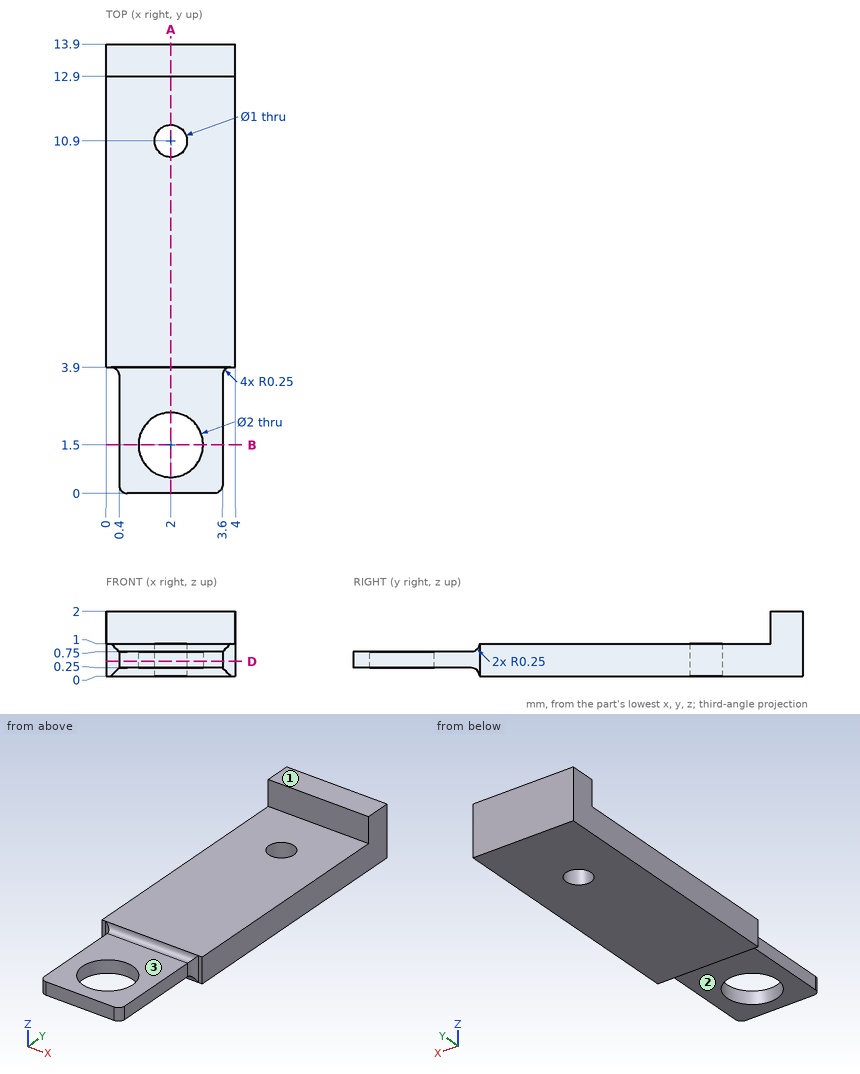
Part print with two shaded views. Sizes in mm from the minimum x, y, z corner. A direction names the side the tool comes from. Round coordinates to 2 decimals unless told otherwise and drop trailing zeros. Order: outer loops, then holes, each group sorted by start corner. A loop starts at its lowest first (then second) coordinate and runs counter-clockwise, first axis right, second up. Notation, with made-up numbers: M 51.5,-13 L 82.5,-13 A17 ccw 82.5,15 Z; hole C -29.75,87 d5. An arc over 180 degrees is marked long. Use CSV: the item, a comma, the result in double quotes. Start each with the question number.
(1) Flat gauge pins, fed straight in: P1, Ø1.2, axis at x = 2, y = 10.5, coming from the +Z side; P2, Ø1, axis at x = 3, y = 1.5, coming from the +Z side; P3, Ø1, axis at x = 1.5, y = 1, coming from the -Z side. Where does each tip first touch, or does it go through?
(2) Cut at A-A on x = 2. State how many separate pieces and enclosed holes the cut face has, then the cut area to 3 significant figures.
(3) Tool access for the marked faces 1, 2 and 3: list every direction of +Z, -Z, +X, -X, +Y, -Y with a clear straight run to the whole face (end or side of a thin tool).
(4) Drill centre lines: probe 1 along Y at (x, z) = (2, 0.65); probe 2 along Z at (x, y) = (3.15, 7); probe 3 along Z at (x, y) = (3.2, 3). Where is each one in solid material? Low to high.
(5) Cut at D-D on z = 0.45. List the corners of the cut face in (x, y).
(6) Cut at B-B on y = 1.5. List the corners of the cut face in (x, z).
Findings:
1,P1,"stops at z = 1"
1,P2,"stops at z = 0.75"
1,P3,"stops at z = 0.25"
2,separate pieces,"3"
2,enclosed holes,"0"
2,area,"11.0 mm^2"
3,face 1,"+Z, +X, -X, +Y, -Y"
3,face 2,"-Z, +X, -X, -Y"
3,face 3,"+Z, +X, -X, -Y"
4,probe 1,"y = 0 to 0.5, 2.5 to 10.4, 11.4 to 13.9"
4,probe 2,"z = 0 to 1"
4,probe 3,"z = 0.25 to 0.75"
5,outline,"M 0,3.9 L 0.15,3.9 A0.25 cw 0.4,3.65 L 0.4,0.25 A0.25 ccw 0.65,0 L 3.35,0 A0.25 ccw 3.6,0.25 L 3.6,3.65 A0.25 cw 3.85,3.9 L 4,3.9 L 4,13.9 L 0,13.9 Z; hole C 2,1.5 d2; hole C 2,10.9 d1"
6,outline,"M 0.4,0.25 L 1,0.25 L 1,0.75 L 0.4,0.75 Z; M 3,0.25 L 3.6,0.25 L 3.6,0.75 L 3,0.75 Z"
